Geometry check sheet. Reference: the model listing, model coordinates, mm. Face numbers are marked on the shaded views. A direction names the side the tool comes from. Round coordinates to 2 decimals unless told otherwise and drop trailing zeros. Write each loop counter-clockwise with the first axis right and the second up, starting at its lowest first coordinate (ties: lowest second). Pieces come first, ordered by that corner, then holes. Notation, with made-up numbers: (40, -15.5) -> (84, -15.5) arc R31 cw to (84, 17.5) -> close; hole circle Ø5 at (-3, 89.25). An arc over 180 degrees is marked (long way). Use a Markdown table: item, result.
```python
from build123d import *

# Parameters (mm, degrees)
BASE_EXTRUSION_DEPTH    = 8
ESQUISSE2_R             = 2.25
ENL_V_MAT_EXTRU_1_DEPTH = 3
CONG_1_R                = 0.3


with BuildPart() as part:
    # Esquisse1 → Base-Extrusion (new body)
    with BuildSketch(Plane.XY):
        with BuildLine():
            Line((0, 0), (10, 0))
            Line((10, 0), (10, 3))
            ThreePointArc((10, 3), (13, 6), (16, 3))
            Line((16, 3), (16, 0))
            Line((16, 0), (18, 0))
            Line((18, 0), (18, 3))
            ThreePointArc((18, 3), (13, 8), (8, 3))
            Line((8, 3), (8, 2))
            Line((8, 2), (0, 2))
            Line((0, 2), (0, 0))
        make_face()
    extrude(amount=BASE_EXTRUSION_DEPTH)

    # Esquisse2 → Enlèv. mat.-Extru.1 (cut, through all)
    with BuildSketch(Plane(origin=(0, 2, 0), x_dir=(-1, 0, 0), z_dir=(0, 1, 0))):
        with Locations((-4, 4)):
            Circle(ESQUISSE2_R)
    extrude(amount=-ENL_V_MAT_EXTRU_1_DEPTH, mode=Mode.SUBTRACT)

    # Congé1
    cong_1_edges = [part.edges().sort_by_distance(p)[0] for p in [
        (8, 2, 4),
    ]]
    fillet(cong_1_edges, radius=CONG_1_R)


solid = part.part
```
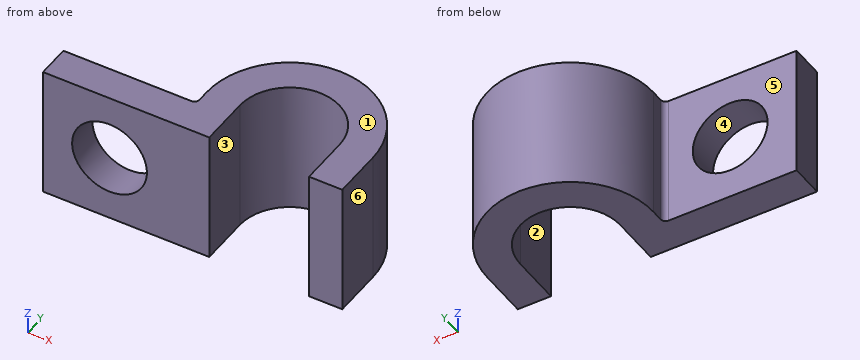
(1) Section check A-A on y = 2.75. Record the cut outline in (x, z).
A:
| item | result |
|---|---|
| outline | (8, 0) -> (10, 0) -> (10, 8) -> (8, 8) -> close; (16, 0) -> (18, 0) -> (18, 8) -> (16, 8) -> close |
(2) Section check D-D on z = 7.5. Record the cut outline in (x, y), plus the area to 3 significant figures.
A:
| item | result |
|---|---|
| outline | (0, 0) -> (10, 0) -> (10, 3) arc R3 cw to (16, 3) -> (16, 0) -> (18, 0) -> (18, 3) arc R5 ccw to (8, 3) -> (8, 2.3) arc R0.3 cw to (7.7, 2) -> (0, 2) -> close |
| area | 53.2 mm2 |
(3) Section check C-C on x = 4. Record the cut outline in (y, z), plus the area to 3 significant figures.
A:
| item | result |
|---|---|
| outline | (0, 0) -> (2, 0) -> (2, 1.75) -> (0, 1.75) -> close; (0, 6.25) -> (2, 6.25) -> (2, 8) -> (0, 8) -> close |
| area | 7.00 mm2 |
(4) Thickness scan on line 1 (X direction, y = 3, z = 4.75); line 2 (Z direction, x = 4, y = 0.9); line 3 (X direction, y = 1, z = 1). Record the ranges inside material, lowest first.
A:
| item | result |
|---|---|
| line 1 | x = 8 to 10, 16 to 18 |
| line 2 | z = 0 to 1.75, 6.25 to 8 |
| line 3 | x = 0 to 10, 16 to 18 |
(5) Access from +Z, -Z, +X, -X, +Y, -Y to the whole of each face (thin tool, end or side, straight path). Record for the marked faces 1 and 2.
A:
| item | result |
|---|---|
| face 1 | +Z, +X, -X, +Y, -Y |
| face 2 | +Z, -Z, -Y |
(6) Section check B-B on z = 4. Record the cut outline in (x, y), plus the area to 3 significant figures.
A:
| item | result |
|---|---|
| outline | (0, 0) -> (1.75, 0) -> (1.75, 2) -> (0, 2) -> close; (6.25, 0) -> (10, 0) -> (10, 3) arc R3 cw to (16, 3) -> (16, 0) -> (18, 0) -> (18, 3) arc R5 ccw to (8, 3) -> (8, 2.3) arc R0.3 cw to (7.7, 2) -> (6.25, 2) -> close |
| area | 44.2 mm2 |
(7) Release check for a two-part mould opening along X. For the marked faces 3, 4, 5 and 6 record: +X half, -X half, draft (parallel to the pull), parting line (faces both ways), or undercut.
A:
| item | result |
|---|---|
| face 3 | undercut |
| face 4 | undercut |
| face 5 | draft |
| face 6 | +X half |
(8) Gauge pin test, flat ends, axial feed: pin 1 Ø1.5 at (y, z) = (6, 3.5) entering from +X; pin 2 Ø1 at (y, z) = (7, 2.5) entering from +X; pin 3 Ø2.5 at (x, z) = (3.5, 2.5) entering from +Y. Record the tip position at first contact, or that the pin passes through.
A:
| item | result |
|---|---|
| pin 1 | stops at x = 17.47 |
| pin 2 | stops at x = 16.57 |
| pin 3 | stops at y = 2 |
